from build123d import *

# Parameters (mm, degrees)
F2_DEPTH = 3
F1_R     = 0.5
F3_DEPTH = 1.5
F4_DEPTH = 1.5
F5_R     = 1.5


with BuildPart() as f2:
    # F0 (on Right) → F2 (new body)
    with BuildSketch(Plane.YZ):
        with BuildLine():
            Line((1.5, 0), (-1.5, 0))
            Line((-1.5, 0), (-1.5, -90))
            ThreePointArc((-1.5, -90), (-9.847457, -110.152543), (-30, -118.5))
            Line((-30, -118.5), (-30, -121.5))
            ThreePointArc((-30, -121.5), (-7.726136, -112.273864), (1.5, -90))
            Line((1.5, -90), (1.5, 0))
        make_face()
    extrude(amount=F2_DEPTH)

    # F1 (on Front) → F3 (cut)
    with BuildSketch(Plane.XZ):
        with Locations((1.5, -1.25)):
            Circle(F1_R)
    extrude(amount=-F3_DEPTH, mode=Mode.SUBTRACT)

    # F1 (on Front) → F4 (cut)
    with BuildSketch(Plane.XZ):
        with Locations((1.5, -1.25)):
            Circle(F1_R)
    extrude(amount=F4_DEPTH, mode=Mode.SUBTRACT)

    # F5
    f5_edges = [f2.edges().sort_by_distance(p)[0] for p in [
        (3, 0, 0),
    ]]
    fillet(f5_edges, radius=F5_R)


solid = f2.part
CAD build for the part. Positions are in the model's coordinates, mm. A direction names the side the tool comes from. Round coordinates to 2 decimals unless told otherwise and drop trailing zeros. Order: outer loops, then holes, each group sorted by start corner. A loop starts at its lowest first (then second) coordinate and runs counter-clockwise, first axis right, second up. Notation, with made-up numbers: (7.5, -31) -> (22.5, -31) arc R28 cw to (22.5, -6) -> close; hole circle Ø10 at (-30, 36.25). An arc over 180 degrees is marked (long way). Write each question's results on one line, items separated by ' | '.
1. 3-axis set-ups, long thin cutter, end or side, ignore diameter. For faces 1 (the face through (1, -1.5, -44)), 2 (the face through (1, -30, -120)): which of +Z, -Z, +X, -X, +Y, -Y reach the whole face in a straight line?
Findings below:
face 1: +Z, +X, -X, -Y | face 2: +Z, -Z, +X, -X, -Y
2. Cut at A-A (x = 2.5). Give the cut face in (y, z).
Findings below:
outline: (-30, -121.5) arc R31.5 ccw to (1.5, -90) -> (1.5, -0.38) -> (-1.5, -0.38) -> (-1.5, -90) arc R28.5 cw to (-30, -118.5) -> close
3. Flat gauge pins, fed straight in: P1, Ø1, axis at x = 1, y = -17, coming from the -Z side; P2, Ø4, axis at y = -2, z = -39, coming from the +X side; P3, Ø1, axis at x = 1, z = -80, coming from the -Y side. Where does each tip first touch, or does it go through?
Findings below:
P1: stops at z = -118.91 | P2: stops at x = 3 | P3: stops at y = -1.5
4. Cut at B-B (z = -38). Give the cut face in (x, y), plus the area to 3 significant figures.
Findings below:
outline: (0, -1.5) -> (3, -1.5) -> (3, 1.5) -> (0, 1.5) -> close | area: 9.00 mm²
5. Wall check: line 1 along Y through (x, z) = (2.4, -75); line 2 along X through (y, z) = (0, -1); line 3 along Y through (x, z) = (1.75, -97). Give the ranges that are in metal, low to high. Write a range as [from, to].
Findings below:
line 1: y = [-1.5, 1.5] | line 2: x = [0, 1.07], [1.93, 2.91] | line 3: y = [-2.37, 0.71]
6. Cut at C-C (y = -4.5). Give the cut face in (x, z).
Findings below:
outline: (0, -108.49) -> (3, -108.49) -> (3, -102.73) -> (0, -102.73) -> close
